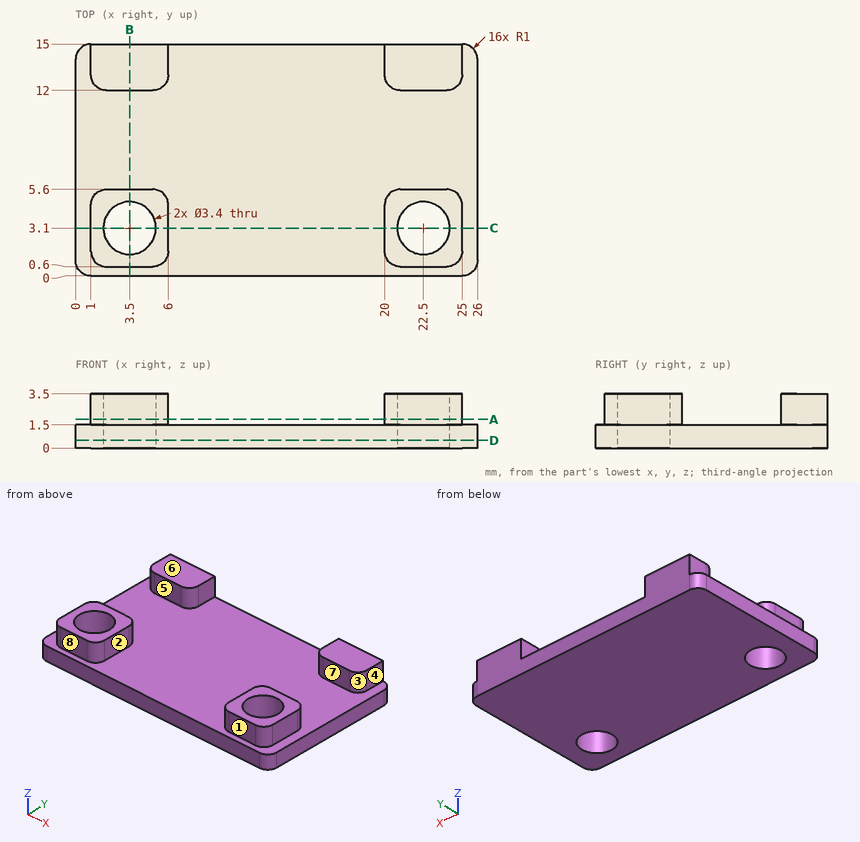
The figure shows three views and two pictorial views of one solid part (mm, origin at its lowest corner). Answer the questions. A direction names the side the tool comes from. Coordinates: 2 decimals unless noted, no trailing zeros. Loops run counter-clockwise (first coordinate to the right, second up) from the corner with the lowest first, then second, coordinate; pieces in that order, holes last.
1) Find section A-A on z = 1.85. Give the number of separate pieces and of enclosed holes in the cut face, then the cut area to 3 significant figures.
2) Find section B-B on x = 3.5. Write down the section's boundary in (y, z).
3) Find section C-C on y = 3.1. Write down the section's boundary in (x, z).
4) Flat-ended cylindrical pins translate along their axes: pin 1 Ø0.6 at (y, z) = (3.5, 3) entering from -X; pin 2 Ø1.5 at (y, z) = (9.5, 2.5) entering from +X; pin 3 Ø1 at (x, z) = (3, 2.5) entering from -Y; pin 4 Ø1 at (y, z) = (3, 2.5) entering from +X. Find the tip coordinate at first contact, or state that the pin passes through.
5) Find the intervals of material crossed by L1, parallel to Y at x = 3.5, z = 1.6; L2, parallel to Y at x = 3.5, z = 0.3; L3, parallel to X at y = 2, z = 1.9, in increasing order.
6) Find section D-D on z = 0.5. Write down the section's boundary in (x, y).
7) Determine the mould class of the marked faces 6, 7 and 8 for opening direction Y: pulls with the +Y half, pulls with the -Y half, needs draft (parallel to the pull), parting line crosses it, or undercut.
8) A tool of negligible diameter and unlimited length cuts with its end or side. For the marked faces 1, 2, 3, 4 and 5, from which of +Z, -Z, +X, -X, +Y, -Y can it reach the whole face along a straight path? Write none if from no direction.
Values:
1. separate pieces: 4
1. enclosed holes: 2
1. area: 59.3 mm2
2. outline: (0, 0) - (1.4, 0) - (1.4, 3.5) - (0.6, 3.5) - (0.6, 1.5) - (0, 1.5) - close; (4.8, 0) - (15, 0) - (15, 3.5) - (12, 3.5) - (12, 1.5) - (5.6, 1.5) - (5.6, 3.5) - (4.8, 3.5) - close
3. outline: (0, 0) - (1.8, 0) - (1.8, 3.5) - (1, 3.5) - (1, 1.5) - (0, 1.5) - close; (5.2, 0) - (20.8, 0) - (20.8, 3.5) - (20, 3.5) - (20, 1.5) - (6, 1.5) - (6, 3.5) - (5.2, 3.5) - close; (24.2, 0) - (26, 0) - (26, 1.5) - (25, 1.5) - (25, 3.5) - (24.2, 3.5) - close
4. pin 1: stops at x = 1
4. pin 2: passes through
4. pin 3: stops at y = 0.6
4. pin 4: stops at x = 25
5. L1: y = 0.6 to 1.4, 4.8 to 5.6, 12 to 15
5. L2: y = 0 to 1.4, 4.8 to 15
5. L3: x = 1 to 2.2, 4.8 to 6, 20 to 21.2, 23.8 to 25
6. outline: (0, 1) arc R1 ccw to (1, 0) - (25, 0) arc R1 ccw to (26, 1) - (26, 14) arc R1 ccw to (25, 15) - (1, 15) arc R1 ccw to (0, 14) - close; hole circle Ø3.4 at (3.5, 3.1); hole circle Ø3.4 at (22.5, 3.1)
7. face 6: needs draft
7. face 7: undercut
7. face 8: pulls with the -Y half
8. face 1: +Z, +X, -X, -Y
8. face 2: +Z, +Y, -Y
8. face 3: +Z, +X
8. face 4: +Z, +X, +Y, -Y
8. face 5: +Z, +X, -X
